Input: dimensioned drawing with shaded views. Units: mm. Origin: part minimum x, y, z. Coordinates: 2 decimals unless noted, no trailing zeros. Order: outer loops, then holes, each group sorted by start corner. A loop starts at its lowest first (then second) coordinate and runs counter-clockwise, first axis right, second up. Notation, with made-up numbers: (27, 69) - (56, 69) arc R36 cw to (56, 105) - close; hole circle Ø9 at (-11, -18). An arc over 180 degrees is marked (long way). Use one line per item in the form item = value. Start each with the question number.
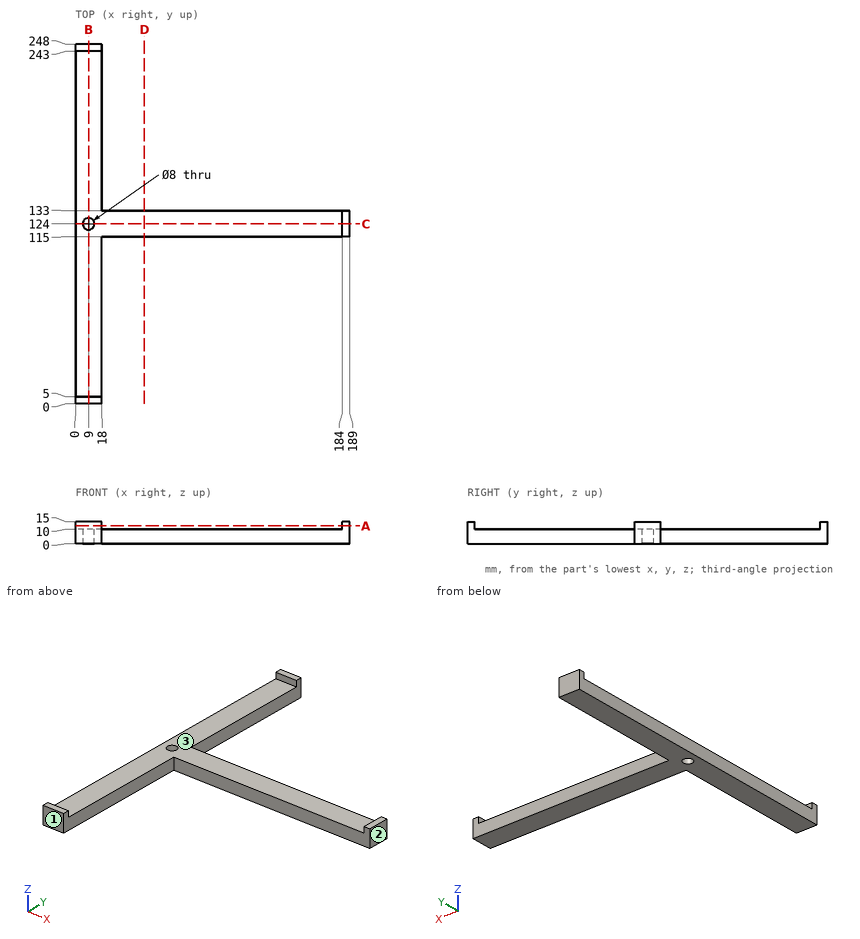
(1) Cut plane A-A on z = 12.25. Return the cut outline in (x, y), plus the area to 3 significant figures.
(2) Cut plane C-C on y = 124. Return the cut outline in (x, z), plus the area to 4 significant figures.
(3) Cut plane B-B on x = 9. Return the cut outline in (y, z).
(4) Draft query along Y for the marked faces 1, 2 and 3. Return one class per face: released by +Y, released by -Y, zero draft, split by the parting line, or undercut.
(5) Cut plane D-D on x = 47.5. Return the cut outline in (y, z), plus the area to 3 significant figures.
(6) Contact query for flat-ended pins moving along their axis: pin 1 Ø7.5 at (y, z) = (29.5, 5.5) entering from +X; pin 2 Ø10.5 at (x, y) = (9, 124) entering from +Z; pin 3 Ø1.5 at (y, z) = (128, 12) entering from -X. Output: stop coordinate, or through.
(7) Material intervals for L1, parallel to Y at x = 9, z = 3.75; L2, parallel to Y at x = 44, z = 6; L3, parallel to Z at x = 100.5, y = 129, sorted ascending. Write a range as from..to.
Check sheet entries:
q1.outline = (0, 0) - (18, 0) - (18, 5) - (0, 5) - close; (0, 243) - (18, 243) - (18, 248) - (0, 248) - close; (184, 115) - (189, 115) - (189, 133) - (184, 133) - close
q1.area = 270 mm^2
q2.outline = (0, 0) - (5, 0) - (5, 10) - (0, 10) - close; (13, 0) - (189, 0) - (189, 15) - (184, 15) - (184, 10) - (13, 10) - close
q2.area = 1,835 mm^2
q3.outline = (0, 0) - (120, 0) - (120, 10) - (5, 10) - (5, 15) - (0, 15) - close; (128, 0) - (248, 0) - (248, 15) - (243, 15) - (243, 10) - (128, 10) - close
q4.face_1 = released by -Y
q4.face_2 = zero draft
q4.face_3 = undercut
q5.outline = (115, 0) - (133, 0) - (133, 10) - (115, 10) - close
q5.area = 180 mm^2
q6.pin_1 = 18
q6.pin_2 = 10
q6.pin_3 = 184
q7.L1 = 0..120, 128..248
q7.L2 = 115..133
q7.L3 = 0..10
